```python
from build123d import *

# Parameters (mm, degrees)
PLATE_START        = -33.55
SKETCH1_R          = 7.25
PLATE_I_DEPTH      = 5
BOLT_START         = -33.75
SKETCH2_R          = 1.7
BOLT_HOLES_DEPTH   = 5.4
COUNTERBORES_START = -33.75
SKETCH3_R          = 3.2
COUNTERBORES_DEPTH = 3.2


with BuildPart() as part:
    # Sketch1 → Plate I (new body)
    with BuildSketch(Plane(origin=(0, 0, 0), x_dir=(0, 0, -1), z_dir=(1, 0, 0)).offset(PLATE_START)):
        with BuildLine():
            Line((-32, 227.975478406), (-32, 288.5))
            ThreePointArc((-32, 288.5), (-30.828427125, 291.328427125), (-28, 292.5))
            Line((-28, 292.5), (0, 292.5))
            ThreePointArc((0, 292.5), (2.828427125, 291.328427125), (4, 288.5))
            Line((4, 288.5), (4, 227.975478406))
            ThreePointArc((4, 227.975478406), (4.49156491, 225.597003504), (5.885714286, 223.608253536))
            ThreePointArc((5.885714286, 223.608253536), (-14, 173.5), (-33.885714286, 223.608253536))
            ThreePointArc((-33.885714286, 223.608253536), (-32.49156491, 225.597003504), (-32, 227.975478406))
        make_face()
        with Locations((-14, 202.5)):
            Circle(SKETCH1_R, mode=Mode.SUBTRACT)
    extrude(amount=PLATE_I_DEPTH)

    # Sketch2 → Bolt holes (cut)
    with BuildSketch(Plane(origin=(0, 0, 0), x_dir=(0, 0, -1), z_dir=(1, 0, 0)).offset(BOLT_START)):
        with Locations((0, 244.5)):
            Circle(SKETCH2_R)
        with Locations((-28, 244.5)):
            Circle(SKETCH2_R)
        with Locations((0, 260.5)):
            Circle(SKETCH2_R)
        with Locations((-28, 260.5)):
            Circle(SKETCH2_R)
        with Locations((-7, 274.5)):
            Circle(SKETCH2_R)
        with Locations((-21, 274.5)):
            Circle(SKETCH2_R)
    extrude(amount=BOLT_HOLES_DEPTH, mode=Mode.SUBTRACT)

    # Sketch3 → Counterbores (cut)
    with BuildSketch(Plane(origin=(0, 0, 0), x_dir=(0, 0, -1), z_dir=(1, 0, 0)).offset(COUNTERBORES_START)):
        with Locations((0, 244.5)):
            Circle(SKETCH3_R)
        with Locations((-28, 244.5)):
            Circle(SKETCH3_R)
        with Locations((0, 260.5)):
            Circle(SKETCH3_R)
        with Locations((-28, 260.5)):
            Circle(SKETCH3_R)
        with Locations((-7, 274.5)):
            Circle(SKETCH3_R)
        with Locations((-21, 274.5)):
            Circle(SKETCH3_R)
    extrude(amount=COUNTERBORES_DEPTH, mode=Mode.SUBTRACT)


solid = part.part
```
The model under review builds one solid part; all positions refer to its coordinate system, in mm. A direction names the side the tool comes from. Coordinates: 2 decimals unless noted, no trailing zeros. Write each loop counter-clockwise with the first axis right and the second up, starting at its lowest first coordinate (ties: lowest second). Pieces come first, ordered by that corner, then holes. Notation, with made-up numbers: (28.25, 3.5) - (63.25, 3.5) arc R25 cw to (63.25, 40.5) - close; hole circle Ø10 at (4, -32). An arc over 180 degrees is marked (long way). Write item = value, one per line.
(1) Mouldability with a two-part tool opening along Y and no side actions: class faces 1 (the face through (-28.55, 221, 14)), 2 (the face through (-31.085, 225.628, -4.478)), 3 (the face through (-29.564, 276.186, 21.221)) as pulls with the +Y half, pulls with the -Y half, needs draft (parallel to the pull), parting line crosses it, or undercut.
Result sheet:
face_1 = needs draft
face_2 = pulls with the +Y half
face_3 = undercut
(2) Consider section C-C, the plane y = 205.5. Give the boundary of the cut face in (x, z), then the cut area to 3 significant figures.
Result sheet:
outline = (-33.55, -14.84) - (-28.55, -14.84) - (-28.55, 7.4) - (-33.55, 7.4) - close; (-33.55, 20.6) - (-28.55, 20.6) - (-28.55, 42.84) - (-33.55, 42.84) - close
area = 222 mm^2
(3) Consider section B-B, the plane y = 274.5. Give the boundary of the cut face in (x, z).
Result sheet:
outline = (-33.55, -4) - (-28.55, -4) - (-28.55, 5.3) - (-30.55, 5.3) - (-30.55, 3.8) - (-33.55, 3.8) - close; (-33.55, 10.2) - (-30.55, 10.2) - (-30.55, 8.7) - (-28.55, 8.7) - (-28.55, 19.3) - (-30.55, 19.3) - (-30.55, 17.8) - (-33.55, 17.8) - close; (-33.55, 24.2) - (-30.55, 24.2) - (-30.55, 22.7) - (-28.55, 22.7) - (-28.55, 32) - (-33.55, 32) - close
(4) Consider section A-A, the plane z = 14. Give the boundary of the cut face in (x, y), then the cut area to 4 significant figures.
Result sheet:
outline = (-33.55, 173.5) - (-28.55, 173.5) - (-28.55, 195.25) - (-33.55, 195.25) - close; (-33.55, 209.75) - (-28.55, 209.75) - (-28.55, 292.5) - (-33.55, 292.5) - close
area = 522.5 mm^2
(5) For P1, Ø4, axis at y = 274.5, z = 21, coming from the -X side; P2, Ø1, axis at x = -32, y = 245.5, coming from the -Z side, all flat-tipped, find the tip position at first contact; note any pin that passes through.
Result sheet:
P1 = -30.55
P2 = -4
(6) Consider section D-D, the plane z = 35. Give the boundary of the cut face in (x, y).
Result sheet:
outline = (-33.55, 182.5) - (-28.55, 182.5) - (-28.55, 222.5) - (-33.55, 222.5) - close
(7) For line 1 (Z direction, x = -31.6, y = 244.5); line 2 (Z direction, x = -30, y = 244.5); line 3 (Y direction, x = -32.45, z = 0), list the stretches that pass through material, from the lowest coordinate up. Write a range as [from, to].
Result sheet:
line_1 = [-4, -3.2], [3.2, 24.8], [31.2, 32]
line_2 = [-4, -1.7], [1.7, 26.3], [29.7, 32]
line_3 = [177.1, 241.3], [247.7, 257.3], [263.7, 292.5]
(8) Machinability: for faces 4 (the face through (-31, 259, -4)), 5 (the face through (-31, 258, 32)), 6 (the face through (-32.071, 271.376, 21.694)), 7 (the face through (-29.564, 276.186, 7.221)), which of the approach directions +Z, -Z, +X, -X, +Y, -Y give a long, thin tool a straight path to every point of the face, cutting with its end or side? Answer none if there is none.
Result sheet:
face_4 = -Z, +X, -X, +Y
face_5 = +Z, +X, -X, +Y
face_6 = -X
face_7 = +X, -X
